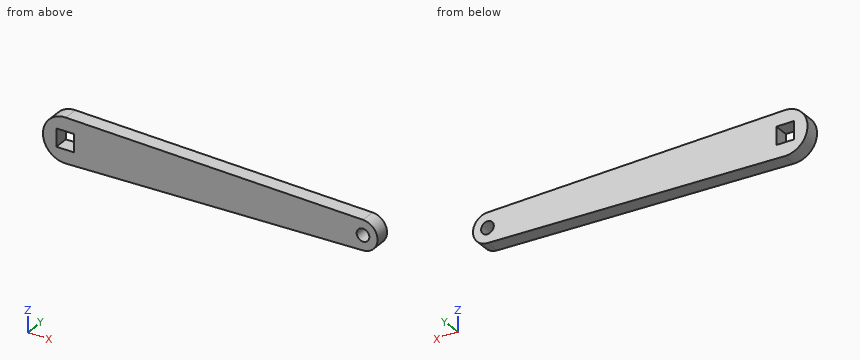
from build123d import *

# Parameters (mm, degrees)
F0_W     = 12
F0_H     = 12
F1_DEPTH = 10
F2_D     = 8.5
F2_DEPTH = 16.5
F2_TIP   = 2.5536576309


with BuildPart() as f1:
    # F0 (on Front) → F1 (new body)
    with BuildSketch(Plane.XZ):
        with BuildLine():
            Line((199.6245300745, 9.9968666721), (0, 14.9953000082))
            ThreePointArc((0, 14.9953000082), (-15.3754699255, 0), (0, -14.9953000082))
            Line((0, -14.9953000082), (199.6245300745, -9.9968666721))
            ThreePointArc((199.6245300745, -9.9968666721), (209.3742167908, 0), (199.6245300745, 9.9968666721))
        make_face()
        with Locations((-0.3754699255, 0)):
            Rectangle(F0_W, F0_H, mode=Mode.SUBTRACT)
    extrude(amount=-F1_DEPTH)

    # F2
    with Locations(Plane.XZ):
        with Locations((199.6245300745, 0)):
            Hole(F2_D / 2, depth=F2_DEPTH)
            with Locations((0, 0, -(F2_DEPTH + F2_TIP / 2))):  # 118° drill point
                Cone(0, F2_D / 2, F2_TIP, mode=Mode.SUBTRACT)


solid = f1.part
Source: CAD feature listing. Evaluate the final solid. Frame: model axes, mm. Coordinates: 2 decimals unless noted, no trailing zeros. Loops run counter-clockwise (first coordinate to the right, second up) from the corner with the lowest first, then second, coordinate; pieces in that order, holes last. Notation, with made-up numbers: M 85,79.25 L 89,79.25 A20 cw 89,109.25 Z; hole C 56.5,-21 d4. An arc over 180 degrees is marked long. Answer in a Markdown table with one row per item.
Q1. Section C-C on z = -13. Return the cut outline in (x, y), plus the area to 3 significant figures.
Answers below:
| item | result |
|---|---|
| outline | M -7.86,0 L 79.69,0 L 79.69,10 L -7.86,10 Z |
| area | 875 mm^2 |
Q2. Section B-B on y = 7.5. Return the cut outline in (x, z), plus the area to 3 significant figures.
Answers below:
| item | result |
|---|---|
| outline | M 0,-15 L 199.62,-10 A10 ccw 199.62,10 L 0,15 A15 ccw long Z; hole M -6.38,-6 L 5.62,-6 L 5.62,6 L -6.38,6 Z; hole C 199.62,0 d8.5 |
| area | 5,310 mm^2 |
Q3. First-contact query: pin 1 (1 mm diameter, centred on y = 2.5, z = -10, fed in from -X); pin 2 (2 mm diameter, centred on x = 62.5, y = 9, fed in from +Z); pin 3 (3 mm diameter, centred on y = 7, z = 2, fed in from -X). Flat tips, straight axial feed; report the tip coordinate or a pass-through.
Answers below:
| item | result |
|---|---|
| pin 1 | stops at x = -11.98 |
| pin 2 | stops at z = 13.46 |
| pin 3 | stops at x = -15.37 |
Q4. Section A-A on z = 0. Return the cut outline in (x, y).
Answers below:
| item | result |
|---|---|
| outline | M -15.38,0 L -6.38,0 L -6.38,10 L -15.38,10 Z; M 5.62,0 L 195.37,0 L 195.37,10 L 5.62,10 Z; M 203.87,0 L 209.37,0 L 209.37,10 L 203.87,10 Z |
Q5. Section D-D on x = 41. Return the cut outline in (y, z), plus the area to 3 significant figures.
Answers below:
| item | result |
|---|---|
| outline | M 0,-13.97 L 10,-13.97 L 10,13.97 L 0,13.97 Z |
| area | 279 mm^2 |
Q6. Ray query, probe 1 along X at (y, z) = (6, -5.5); probe 2 along X at (y, z) = (3.5, 1); probe 3 along Z at (x, y) = (11.5, 3.75). Return the intervals inside material, ascending. Write a range as from..to.
Answers below:
| item | result |
|---|---|
| probe 1 | x = -14.33..-6.38, 5.62..207.73 |
| probe 2 | x = -15.34..-6.38, 5.62..195.49, 203.76..209.32 |
| probe 3 | z = -14.71..14.71 |
